Design review of the part built by this model. Coordinates are the model's own, in mm. Face numbers are marked on the shaded views. A direction names the side the tool comes from. Give positions to 0.01 mm unless a question says otherwise; leave off trailing zeros. Order: outer loops, then holes, each group sorted by start corner. A loop starts at its lowest first (then second) coordinate and runs counter-clockwise, first axis right, second up. Notation, with made-up numbers: (-21.5, 31) -> (-17.5, 31) arc R17 ccw to (-17.5, 63) -> close; hole circle Ø9 at (-28, 79.25). An arc over 180 degrees is marked (long way). Return JSON: item names as keys, results as strings.
```python
from build123d import *

# Parameters (mm, degrees)
IZIM1_R                     = 4.45
Y_KSEKLIK_EKSTR_ZYON1_DEPTH = 5.6
IZIM2_R                     = 0.85
IZIM2_R_2                   = 1.08184978
Y_KSEKLIK_EKSTR_ZYON2_DEPTH = 2.3
DAIRESEL_KAPLAMA1_COUNT     = 4
IZIM3_R                     = 2.5
KES_EKSTR_ZYON1_DEPTH       = 1.05
IZIM4_R                     = 4.65
IZIM4_R_2                   = 3.35
KES_EKSTR_ZYON2_DEPTH       = 1.05
IZIM5_R                     = 1.5
KES_EKSTR_ZYON3_DEPTH       = 7.05
IZIM6_R                     = 2.68
KES_EKSTR_ZYON4_DEPTH       = 3.5
KES_EKSTR_ZYON5_DEPTH       = 3.5
DAIRESEL_KAPLAMA2_COUNT     = 24


with BuildPart() as part:
    # Çizim1 → Yükseklik-Ekstrüzyon1 (new body)
    with BuildSketch(Plane(origin=(0, 0, 0), x_dir=(1, 0, 0), z_dir=(0, 1, 0))):
        with Locations(Location((0, 0, 0), (0, 0, 270))):
            Circle(IZIM1_R)
    extrude(amount=Y_KSEKLIK_EKSTR_ZYON1_DEPTH)

    # Çizim2 → Yükseklik-Ekstrüzyon2 (add)
    with BuildSketch(Plane(origin=(0, 5.6, 0), x_dir=(1, 0, 0), z_dir=(0, 1, 0))):
        with BuildLine():
            Line((0, 4.69), (0, -4.69))
            Line((0, -4.69), (-4.520042194, -4.69))
            Line((-4.520042194, -4.69), (-4.783580891, -4.426461303))
            ThreePointArc((-4.783580891, -4.426461303), (-5.337293558, -4.147310093), (-5.949896194, -4.051179314))
            Line((-5.949896194, -4.051179314), (-7.379896194, -4.051179314))
            Line((-7.379896194, -4.051179314), (-16.5, -1.945637445))
            ThreePointArc((-16.5, -1.945637445), (-18.445637445, 0), (-16.5, 1.945637445))
            Line((-16.5, 1.945637445), (-7.379896194, 4.051179314))
            Line((-7.379896194, 4.051179314), (-5.949896194, 4.051179314))
            ThreePointArc((-5.949896194, 4.051179314), (-5.337293558, 4.147310093), (-4.783580891, 4.426461303))
            Line((-4.783580891, 4.426461303), (-4.520042194, 4.69))
            Line((-4.520042194, 4.69), (0, 4.69))
        make_face()
        with Locations(Location((-16.5, 0, 0), (0, 0, 270))):
            Circle(IZIM2_R, mode=Mode.SUBTRACT)
        with Locations(Location((-13.5, 0, 0), (0, 0, 270))):
            Circle(IZIM2_R, mode=Mode.SUBTRACT)
        with Locations(Location((-10.5, 0, 0), (0, 0, 270))):
            Circle(IZIM2_R, mode=Mode.SUBTRACT)
        with Locations(Location((-7.5, 0, 0), (0, 0, 270))):
            Circle(IZIM2_R_2, mode=Mode.SUBTRACT)
    y_kseklik_ekstr_zyon2 = extrude(amount=-Y_KSEKLIK_EKSTR_ZYON2_DEPTH)

    # Dairesel Kaplama1: Yükseklik-Ekstrüzyon2 ×4 about axis
    dairesel_kaplama1_axis = Axis((0, 0, 0), (0, 1, 0))
    for i in range(1, DAIRESEL_KAPLAMA1_COUNT):
        add(y_kseklik_ekstr_zyon2.rotate(dairesel_kaplama1_axis, i * 360 / DAIRESEL_KAPLAMA1_COUNT))

    # Çizim3 → Kes-Ekstrüzyon1 (cut)
    with BuildSketch(Plane(origin=(0, 5.6, 0), x_dir=(1, 0, 0), z_dir=(0, 1, 0))):
        with Locations(Location((0, 0, 0), (0, 0, 270))):
            Circle(IZIM3_R)
    extrude(amount=-KES_EKSTR_ZYON1_DEPTH, mode=Mode.SUBTRACT)

    # Çizim4 → Kes-Ekstrüzyon2 (cut)
    with BuildSketch(Plane(origin=(0, 4.55, 0), x_dir=(1, 0, 0), z_dir=(0, 1, 0))):
        with Locations(Location((0, 0, 0), (0, 0, 270))):
            Circle(IZIM4_R)
        with Locations(Location((0, 0, 0), (0, 0, 270))):
            Circle(IZIM4_R_2, mode=Mode.SUBTRACT)
    extrude(amount=KES_EKSTR_ZYON2_DEPTH, mode=Mode.SUBTRACT)

    # Çizim5 → Kes-Ekstrüzyon3 (cut)
    with BuildSketch(Plane(origin=(0, 4.55, 0), x_dir=(1, 0, 0), z_dir=(0, 1, 0))):
        with Locations(Location((0, 0, 0), (0, 0, 270))):
            Circle(IZIM5_R)
    extrude(amount=-KES_EKSTR_ZYON3_DEPTH, mode=Mode.SUBTRACT)

    # Çizim6 → Kes-Ekstrüzyon4 (cut)
    with BuildSketch(Plane.XZ):
        with Locations(Location((0, 0, 0), (0, 0, 270))):
            Circle(IZIM6_R)
    extrude(amount=-KES_EKSTR_ZYON4_DEPTH, mode=Mode.SUBTRACT)

    # Çizim7 → Kes-Ekstrüzyon5 (cut)
    with BuildSketch(Plane.XZ.offset(-3.5)):
        with BuildLine():
            Line((-2.357417444, 1.923535533), (-2.484485613, 1.756341991))
            Line((-2.484485613, 1.756341991), (-2.274980692, 1.416637869))
            ThreePointArc((-2.274980692, 1.416637869), (-2.117608163, 1.642600277), (-1.937879889, 1.851221633))
            Line((-1.937879889, 1.851221633), (-2.357417444, 1.923535533))
        make_face()
    kes_ekstr_zyon5 = extrude(amount=KES_EKSTR_ZYON5_DEPTH, mode=Mode.SUBTRACT)

    # Dairesel Kaplama2: Kes-Ekstrüzyon5 ×24 about axis
    dairesel_kaplama2_axis = Axis((0, 0, 0), (0, 1, 0))
    for i in range(1, DAIRESEL_KAPLAMA2_COUNT):
        add(kes_ekstr_zyon5.rotate(dairesel_kaplama2_axis, i * 360 / DAIRESEL_KAPLAMA2_COUNT), mode=Mode.SUBTRACT)


solid = part.part
```
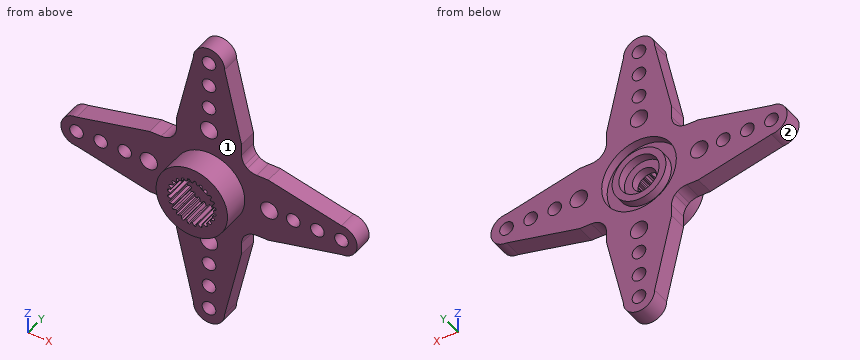
Item 1: Wall thickness on L1, parallel to Z at x = 13.5, y = 4.7; L2, parallel to X at y = 1.55, z = -2; L3, parallel to Z at x = 7.5, y = 4.7: over which ranges is each line inside the solid? List them lowest first. Write a range as [from, to].
Result set:
{"L1": "z = [-2.64, -0.85], [0.85, 2.64]", "L2": "x = [-3.98, -1.86], [1.84, 3.98]", "L3": "z = [-4.02, -1.08], [1.08, 4.02]"}
Item 2: Add section B-B (x = -13.5). Give the boundary of the cut face in (y, z).
Result set:
{"outline": "(3.3, -2.64) -> (5.6, -2.64) -> (5.6, -0.85) -> (3.3, -0.85) -> close; (3.3, 0.85) -> (5.6, 0.85) -> (5.6, 2.64) -> (3.3, 2.64) -> close"}
Item 3: Add section C-C (z = 13.5). Give the boundary of the cut face in (x, y), plus the area to 3 significant figures.
Result set:
{"outline": "(-2.64, 3.3) -> (-0.85, 3.3) -> (-0.85, 5.6) -> (-2.64, 5.6) -> close; (0.85, 3.3) -> (2.64, 3.3) -> (2.64, 5.6) -> (0.85, 5.6) -> close", "area": "8.23 mm^2"}
Item 4: Add section D-D (x = 5.5). Give the boundary of the cut face in (y, z).
Result set:
{"outline": "(3.3, -4.1) -> (5.6, -4.1) -> (5.6, 4.1) -> (3.3, 4.1) -> close"}
Item 5: For pin 1 (2 mm diameter, centred on x = 8, y = 3.5, fed in from +Z); pin 2 (0.7 mm diameter, centred on y = 5, z = 6.5, fed in from +X); pin 3 (1.1 mm diameter, centred on x = -7, y = 4, fed in from -Z); pin 4 (2.5 mm diameter, centred on x = 0, z = 16.5, fed in from +Y), all flat-tipped, find the tip position at first contact; note any pin that passes through.
Result set:
{"pin 1": "stops at z = 4.05", "pin 2": "stops at x = 4.05", "pin 3": "stops at z = -4.05", "pin 4": "stops at y = 5.6"}
Item 6: Add section A-A (y = 5). Give the number of separate pieces and of enclosed holes in the cut face, plus the area to 3 significant figures.
Result set:
{"separate pieces": "2", "enclosed holes": "18", "area": "325 mm^2"}
Item 7: Machinability: for the marked faces 1 and 2, which of the approach directions +Z, -Z, +X, -X, +Y, -Y give a long, thin tool a straight path to every point of the face, cutting with its end or side? Answer none if there is none.
Result set:
{"face 1": "-Y", "face 2": "-X, +Y, -Y"}
